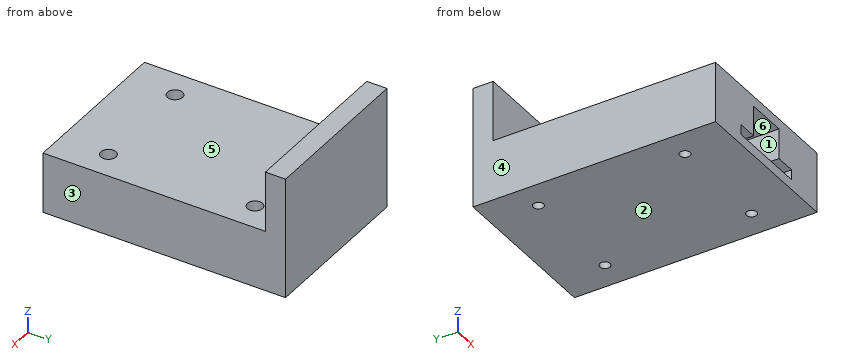
from build123d import *

# Parameters (mm, degrees)
F0_W     = 203.2
F0_H     = 76.2
F1_DEPTH = 304.8
F2_W     = 203.2
F2_H     = 25.4
F3_DEPTH = 76.2
F4_R     = 9.525
F4_R_2   = 6.35
F5_DEPTH = 19.05
F6_DEPTH = 76.201


with BuildPart() as f1:
    # F0 (on Front) → F1 (new body)
    with BuildSketch(Plane.XZ):
        with Locations((0, -38.1)):
            Rectangle(F0_W, F0_H)
        Polygon((-50.8, -63.5), (-50.8, -50.8), (-25.4, -50.8), (-25.4, -12.7), (25.4, -12.7), (25.4, -50.8), (50.8, -50.8), (50.8, -63.5), align=None, mode=Mode.SUBTRACT)
    extrude(amount=F1_DEPTH)

    # F2 (on Top) → F3 (join, symmetric)
    with BuildSketch(Plane.XY):
        with Locations((0, -12.7)):
            Rectangle(F2_W, F2_H)
    extrude(amount=F3_DEPTH, both=True)

    # F4 (on Top) → F5 (cut)
    with BuildSketch(Plane.XY):
        with Locations((-66.675, -60.325)):
            Circle(F4_R)
        with Locations((-66.675, -60.325)):
            Circle(F4_R_2, mode=Mode.SUBTRACT)
        with Locations((66.675, -60.325)):
            Circle(F4_R)
        with Locations((66.675, -60.325)):
            Circle(F4_R_2, mode=Mode.SUBTRACT)
        with Locations((66.675, -244.475)):
            Circle(F4_R)
        with Locations((66.675, -244.475)):
            Circle(F4_R_2, mode=Mode.SUBTRACT)
        with Locations((-66.675, -244.475)):
            Circle(F4_R)
        with Locations((-66.675, -244.475)):
            Circle(F4_R_2, mode=Mode.SUBTRACT)
    extrude(amount=-F5_DEPTH, mode=Mode.SUBTRACT)

    # F6 (cut, through all): faces of the model
    f6_faces = [f1.faces().sort_by_distance(p)[0] for p in [
        (-66.675, -60.325, 0),
        (66.675, -60.325, 0),
        (-66.675, -244.475, 0),
        (66.675, -244.475, 0),
    ]]
    extrude(f6_faces, amount=-F6_DEPTH, mode=Mode.SUBTRACT)


solid = f1.part
Can you work these out from the model? Positions are in its coordinate system, mm. Face numbers are marked on the shaded views. A direction names the side the tool comes from. Round coordinates to 2 decimals unless told otherwise and drop trailing zeros. Write each loop counter-clockwise with the first axis right and the second up, starting at its lowest first coordinate (ties: lowest second). Pieces come first, ordered by that corner, then holes. Notation, with made-up numbers: (-36.5, 24) - (2.5, 24) arc R24 cw to (2.5, 48) - close; hole circle Ø2 at (13, 31.25). An arc over 180 degrees is marked (long way). Write each question's results on one line, items separated by ' | '. Start each with the question number.
1) Suppose I cut it at C-C (z = -31). List the corners of the cut face in (x, y) for me (3 decimals), and give its area (3 significant figures).
2) Suppose I cut it at B-B (x = -30). List the corners of the cut face in (y, z) for me.
3) We'd pull the mould along Z, two halves only. Please class the marked faces 1, 2 and 3: released by +Z, released by -Z, zero draft, split by the parting line, or undercut.
4) Which directions (+Z, -Z, +X, -X, +Y, -Y) give clear straight access to the entire face, cutting with the end or side of a thin tool? Please do the marked faces 4, 5 and 6.
5) For pin 1 Ø1 at (x, z) = (12.5, 26.5) entering from -Y; pin 2 Ø11.5 at (x, y) = (66.675, -60.325) entering from -Z; pin 3 Ø6 at (x, y) = (-32.5, -43.5) entering from +Z; pin 4 Ø14.5 at (x, y) = (-66.675, -60.325) entering from +Z, each with a flat end and sliding along its axis, tell me the tip position at first contact or that it passes through.
6) Suppose I cut it at D-D (z = 38). List the corners of the cut face in (x, y) for me.
7) Please list where these lines run through material, in increasing order: line 1 (Z direction, x = -5.5, y = -250); line 2 (X direction, y = -116, z = -20.5); line 3 (Y direction, x = -22, z = 4).
8) Suppose I cut it at A-A (y = -74). List the corners of the cut face in (x, z) for me, and give its area (3 significant figures).
Here are the results:
1) outline: (-101.6, -304.8) - (-25.4, -304.8) - (-25.4, -25.4) - (25.4, -25.4) - (25.4, -304.8) - (101.6, -304.8) - (101.6, 0) - (-101.6, 0) - close; hole circle Ø12.7 at (-66.675, -244.475); hole circle Ø12.7 at (-66.675, -60.325); hole circle Ø12.7 at (66.675, -244.475); hole circle Ø12.7 at (66.675, -60.325) | area: 47,200 mm2
2) outline: (-304.8, -76.2) - (0, -76.2) - (0, 76.2) - (-25.4, 76.2) - (-25.4, 0) - (-304.8, 0) - (-304.8, -50.8) - (-25.4, -50.8) - (-25.4, -63.5) - (-304.8, -63.5) - close
3) face 1: undercut | face 2: released by -Z | face 3: zero draft
4) face 4: +Z, -Z, -X, +Y, -Y | face 5: +Z, +X, -X, -Y | face 6: -Y
5) pin 1: stops at y = -25.4 | pin 2: passes through | pin 3: stops at z = 0 | pin 4: stops at z = -19.05
6) outline: (-101.6, -25.4) - (101.6, -25.4) - (101.6, 0) - (-101.6, 0) - close
7) line 1: z = -76.2 to -63.5, -12.7 to 0 | line 2: x = -101.6 to -25.4, 25.4 to 101.6 | line 3: y = -25.4 to 0
8) outline: (-101.6, -76.2) - (101.6, -76.2) - (101.6, 0) - (-101.6, 0) - close; hole (-50.8, -63.5) - (50.8, -63.5) - (50.8, -50.8) - (25.4, -50.8) - (25.4, -12.7) - (-25.4, -12.7) - (-25.4, -50.8) - (-50.8, -50.8) - close | area: 12,300 mm2
